Autodesk Inventor part; units mm, degrees
ref_plane "YZ Plane" through (0, 0, 0) normal (1, 0, 0) x (0, 1, 0)
ref_plane "XZ Plane" through (0, 0, 0) normal (0, 1, 0) x (-1, 0, 0)
ref_plane "XY Plane" through (0, 0, 0) normal (0, 0, 1) x (1, 0, 0)
sketch "Sketch1" plane through (0, 0, 0) normal (1, 0, 0) x (0, 1, 0)
  line L0 (0, 35) -> (0, -35)
  line L1 (-35, 0) -> (35, 0)
  line L2 (-25, -25) -> (25, -25)
  line L3 (25, -25) -> (25, 25)
  line L4 (25, 25) -> (-25, 25)
  line L5 (-25, 25) -> (-25, -25)
  line L6 (-25, -25) -> (25, 25) construction
  line L7 (25, -25) -> (-25, 25) construction
  point P0 (0, 0)
  dimension "d1" = 50
  dimension "d2" = 50
extrude "Base" add sketch "Sketch1" along normal mid plane 54
sketch "Sketch2" plane through (27, 0, 0) normal (1, 0, 0) x (0, 0, -1)
  line L0 (-35, 0) -> (35, 0) construction
  line L1 (25, -25) -> (25, 25) construction
  point P0 (0, 0)
  point P1 (5, 0)
  dimension "d5" = 20
hole "Hole_Wheel" at (27, 0, -5) direction (-1, 0, 0) diameter 16 end through all
sketch "Sketch3" plane through (27, 25, -25) normal (0, 0, -1) x (-1, 0, 0)
  line L0 (54, -33) -> (0, -33) construction
  line L1 (54, -17) -> (0, -17) construction
  line L2 (54, 0) -> (0, 0) construction
  line L3 (0, -50) -> (0, 0) construction
  line L4 (0, -50) -> (54, -50) construction
  line L5 (54, 0) -> (54, -50) construction
  line L6 (54, -50) -> (54, 0)
  line L7 (54, -25) -> (0, -25) construction
  line L8 (54, -50) -> (0, -50)
  line L9 (27, -50) -> (27, 0) construction
  line L10 (54, 0) -> (0, 0)
  point P0 (27, -25)
  point P1 (44.5, -25)
  point P2 (9.5, -25)
  point P3 (27, -25)
  dimension "d13" = 35
hole "Hole_Wheel_Fix" at (-17.5, 0, -25) at (17.5, 0, -25) at (0, 0, -25) direction (0, 0, 1) diameter 4.459 end up to surface countersink diameter 11.5 countersink angle 90
sketch "Sketch4" plane through (-27, -25, 25) normal (0, 0, 1) x (1, 0, 0)
  line L0 (54, 50) -> (54, 0) construction
  line L1 (0, 0) -> (0, 50) construction
  line L2 (0, 50) -> (54, 50) construction
  line L3 (0, 0) -> (54, 0) construction
  line L4 (54, 0) -> (54, 50) construction
  line L5 (52, 52) -> (0, 0) construction
  line L6 (54, 0) -> (0, 0) construction
  line L7 (52, -2) -> (0, 50) construction
  point P0 (27, 25)
  point P1 (27, 25)
hole "ConnectionPipe" at (0, 0, 25) direction (0, 0, -1) diameter 20 depth 15 tip angle 118
chamfer "Chamfer1" distance 10 angle 45 4 edges at (0, 25, -25) (0, -25, -25) (0, 25, 25) (0, -25, 25)
chamfer "Chamfer2" distance 1 angle 45 2 edges at (-27, 0, 3) (27, 0, 3)
properties part number "10-004-ACTR-FIX" material "Stainless Steel"
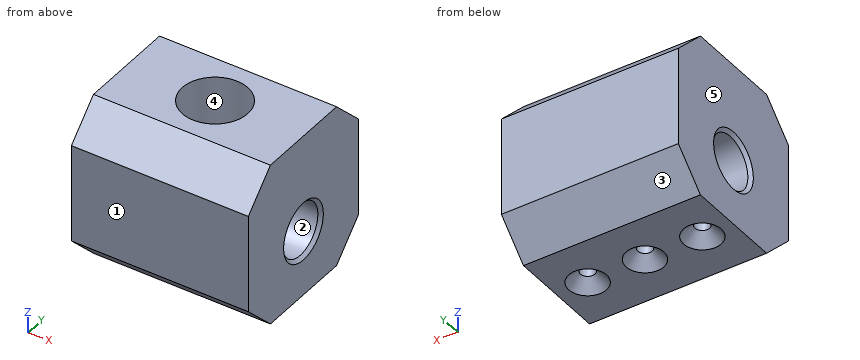
Could you check a few things on this model? Use its own coordinates, in mm. Face numbers are marked on the shaded views. A direction names the side the tool comes from. Coordinates: 2 decimals unless noted, no trailing zeros. Loops run counter-clockwise (first coordinate to the right, second up) from the corner with the lowest first, then second, coordinate; pieces in that order, holes last.
1. For the marked faces 4 and 5, which set-ups out of +Z, -Z, +X, -X, +Y, -Y let a thin tool reach every point of the face, with its end or its side?
2. Imagine slicing it at A-A (z = -20). Please give me the cut outline in (x, y), and give its area (3 significant figures).
3. I need wall thicknesses on L1, parallel to X at y = 0, z = -17; L2, parallel to Y at x = -8.5, z = -5; L3, parallel to Z at x = 1.5, y = -6. Which ranges of each line are inside material? Lowest first, please.
4. Imagine slicing it at B-B (y = 18). Please give me the cut outline in (x, z), and give its area (3 significant figures).
5. Imagine slicing it at C-C (y = -17.5). Please give me the cut outline in (x, z).
6. For P1, Ø4, axis at x = -17.5, y = 0, coming from the -Z side; P2, Ø2, axis at y = 3.5, z = 0, coming from the +X side; P3, Ø5, axis at x = 0, y = 0, coming from the +Z side, each with a flat end and sliding along its axis, tell me the tip position at first contact or that it passes through.
7. We'd pull the mould along Z, two halves only. Please class the marked faces 1, 2 and 3: released by +Z, released by -Z, zero draft, split by the parting line, or undercut.
Computed values:
1. face 4: +Z
1. face 5: +Z, -Z, -X, +Y, -Y
2. outline: (-27, -20) - (27, -20) - (27, 20) - (-27, 20) - close; hole circle Ø4.46 at (-17.5, 0); hole circle Ø4.46 at (0, 0); hole circle Ø4.46 at (17.5, 0)
2. area: 2,110 mm2
3. L1: x = -27 to -19.73, -15.27 to -2.23, 2.23 to 15.27, 19.73 to 27
3. L2: y = -25 to -8, 8 to 25
3. L3: z = -25 to -10.29, 0.29 to 7.71
4. outline: (-27, -22) - (27, -22) - (27, 22) - (-27, 22) - close
4. area: 2,380 mm2
5. outline: (-27, -22.5) - (27, -22.5) - (27, 22.5) - (-27, 22.5) - close
6. P1: stops at z = 2.75
6. P2: passes through
6. P3: stops at z = 5.49
7. face 1: zero draft
7. face 2: undercut
7. face 3: released by -Z
